The listing builds one solid part. Answer for the finished solid, in the listing's coordinates (mm). A direction names the side the tool comes from. Give positions to 0.01 mm unless a question says otherwise; leave off trailing zeros. Write each loop counter-clockwise with the first axis right and the second up, starting at its lowest first coordinate (ties: lowest second). Pieces come first, ordered by that corner, then holes. Notation, with made-up numbers: (14, -31.5) - (34, -31.5) arc R18 cw to (34, 1.5) - close; hole circle Ø5 at (-14.75, -34). An arc over 180 degrees is marked (long way). Return JSON: item names as keys, results as strings.
from build123d import *

# Parameters (mm, degrees)
BOSS_EXTRUDE1_DEPTH = 21.59
SKETCH2_R           = 3.175
BOSS_EXTRUDE3_DEPTH = 2.54
BOSS_EXTRUDE4_START = 3.81
SKETCH3_R           = 3.175
BOSS_EXTRUDE4_DEPTH = 3.81
SKETCH4_R           = 3.175
BOSS_EXTRUDE5_DEPTH = 5.08


with BuildPart() as part:
    # Sketch1 → Boss-Extrude1 (new body)
    with BuildSketch(Plane.XY):
        with BuildLine():
            Line((-621.150306902, 90.224895892), (-621.092144063, 94.034451914))
            Line((-621.092144063, 94.034451914), (-629.598897849, 94.164329766))
            ThreePointArc((-629.598897849, 94.164329766), (-632.210560309, 95.031876848), (-634.47123768, 96.601194079))
            ThreePointArc((-634.47123768, 96.601194079), (-637.543945735, 103.811741783), (-634.252545404, 110.925124722))
            Line((-634.252545404, 110.925124722), (-640.60180544, 111.022062787))
            Line((-640.60180544, 111.022062787), (-640.914721516, 90.52665139))
            Line((-640.914721516, 90.52665139), (-621.150306902, 90.224895892))
        make_face()
    extrude(amount=-BOSS_EXTRUDE1_DEPTH)

    # Sketch2 → Boss-Extrude3 (add)
    # profile 1 of 2: a face of its own
    with BuildSketch(Plane(origin=(0, 0, -19.05), x_dir=(-1, 0, 0), z_dir=(0, 0, -1))):
        with BuildLine():
            Line((620.837390826, 110.72030729), (621.056083102, 96.396376647))
            Line((621.056083102, 96.396376647), (634.47123768, 96.601194079))
            ThreePointArc((634.47123768, 96.601194079), (637.543945735, 103.811741783), (634.252545404, 110.925124722))
            Line((634.252545404, 110.925124722), (620.837390826, 110.72030729))
        make_face()
        with Locations(Location((627.893070479, 103.664395923, 0), (0, 0, 180))):
            Circle(SKETCH2_R, mode=Mode.SUBTRACT)
    # profile 2 of 2: a face of its own
    with BuildSketch(Plane(origin=(0, 0, -19.05), x_dir=(-1, 0, 0), z_dir=(0, 0, -1))):
        with BuildLine():
            Line((621.056083102, 96.396376647), (621.092144063, 94.034451914))
            Line((621.092144063, 94.034451914), (629.598897849, 94.164329766))
            ThreePointArc((629.598897849, 94.164329766), (632.210560309, 95.031876848), (634.47123768, 96.601194079))
            Line((634.47123768, 96.601194079), (621.056083102, 96.396376647))
        make_face()
    extrude(amount=BOSS_EXTRUDE3_DEPTH)

    # Sketch3 → Boss-Extrude4 (add)
    with BuildSketch(Plane.XY.offset(BOSS_EXTRUDE4_START)):
        Polygon((-640.60180544, 111.022062787), (-620.837390826, 110.72030729), (-621.150306902, 90.224895892), (-640.914721516, 90.52665139), align=None)
        with Locations((-627.893070479, 103.664395923)):
            Circle(SKETCH3_R, mode=Mode.SUBTRACT)
    extrude(amount=-BOSS_EXTRUDE4_DEPTH)

    # Sketch4 → Boss-Extrude5 (add)
    with BuildSketch(Plane(origin=(-1.009584834, 97.256608571, -1.08885119), x_dir=(0.9999461323694532, 0.010378769561310733, -0.00011619709707159695), z_dir=(-0.010379419992088095, 0.9998834703189057, -0.011194347843893974))):
        Polygon((-726.19647196, 95.087156462), (-619.816577451, -34.574539021), (-600.038415617, -18.347705324), (-706.418310126, 111.313990158), align=None)
        with Locations(Location((-713.367901644, 95.087156462, 0), (0, 0, 270))):
            Circle(SKETCH4_R, mode=Mode.SUBTRACT)
        with Locations(Location((-609.755864614, -16.672880145, 0), (0, 0, 270))):
            Circle(SKETCH4_R, mode=Mode.SUBTRACT)
    extrude(amount=-BOSS_EXTRUDE5_DEPTH)


solid = part.part
Item 1: A cutting plane is placed at C-C on x = -690. Determine the outline of the cut face in (y, z), then the cut area to 3 significant figures.
Answer below:
{"outline": "(84.02, -91.13) - (89.1, -91.12) - (89.55, -50.79) - (84.47, -50.8) - close", "area": "205 mm²"}
Item 2: For faces 1 (the face through (-631.065, 103.804, 1.932)), 2 (the face through (-631, 101, 0)), determine the directions among +Z, -Z, +X, -X, +Y, -Y from which every point of the face is accessible in a straight line to the end or side of a thin tool.
Answer below:
{"face 1": "+Z, -Z", "face 2": "+X"}
Item 3: A cutting plane is placed at B-B on z = -3.5. Determine the outline of the cut face in (x, y), then the cut area to 3 significant figures.
Answer below:
{"outline": "(-651.2, 90.48) - (-651.19, 85.4) - (-618.1, 85.74) - (-618.11, 90.82) - (-621.14, 90.79) - (-621.09, 94.03) - (-629.6, 94.16) arc R9.65 cw to (-634.25, 110.93) - (-640.6, 111.02) - (-640.91, 90.59) - close", "area": "316 mm²"}
Item 4: A cutting plane is placed at D-D on z = -73. Determine the outline of the cut face in (x, y), then the cut area to 3 significant figures.
Answer below:
{"outline": "(-708.22, 84.03) - (-675.13, 84.37) - (-675.13, 89.45) - (-708.22, 89.11) - close", "area": "168 mm²"}
Item 5: A cutting plane is placed at A-A on y = 98.5. Determine the outline of the cut face in (x, z), then the cut area to 3 significant figures.
Answer below:
{"outline": "(-640.79, -21.59) - (-621.02, -21.59) - (-621.02, -19.05) - (-636.05, -19.05) - (-636.05, 0) - (-621.02, 0) - (-621.02, 3.81) - (-640.79, 3.81) - close", "area": "216 mm²"}
Item 6: Flat-ended cylindrical pins translate along their axes: P1, Ø10, axis at y = 97.5, z = -14.5, coming from the +X side; P2, Ø1, axis at x = -655, y = 92.5, coming from the +Z side; P3, Ø10, axis at x = -627.89, y = 103.66, coming from the +Z side; P4, Ø10, axis at x = -636, y = 89, coming from the +Z side. Find the tip coordinate at first contact, or state that the pin passes through.
Answer below:
{"P1": "stops at x = -621.01", "P2": "passes through", "P3": "stops at z = 3.81", "P4": "stops at z = 21.11"}
Item 7: The mould has two halves that part along Y. Classify faces 3 (the face through (-631, 101, 3.81)), 4 (the face through (-631.065, 103.525, -20.302)): +Y half, -Y half, draft (parallel to the pull), parting line (faces both ways), or undercut.
Answer below:
{"face 3": "draft", "face 4": "undercut"}
Item 8: Consider L1, parallel to Z at x = -623, y = 94.75; L2, parallel to Z at x = -630, y = 92; L3, parallel to Y at x = -647.5, z = -38.5. Determine where each line is inside the solid, lowest interval first.
Answer below:
{"L1": "z = -21.59 to -19.05, 0 to 3.81", "L2": "z = -21.59 to 3.81", "L3": "y = 85.05 to 90.13"}
